```python
from build123d import *

# Parameters (mm, degrees)
SKETCH1_R           = 6
BOSS_EXTRUDE1_DEPTH = 3
SKETCH2_R           = 5.5
BOSS_EXTRUDE2_DEPTH = 0.5
SKETCH3_R           = 6
BOSS_EXTRUDE3_DEPTH = 5
SKETCH4_R           = 1.15
CUT_EXTRUDE1_DEPTH  = 5
SKETCH5_R           = 0.3
BOSS_EXTRUDE4_DEPTH = 5
FILLET1_R           = 0.1
CHAMFER1_SIZE       = 0.05


with BuildPart() as part:
    # Sketch1 → Boss-Extrude1 (new body)
    with BuildSketch(Plane(origin=(0, 0, 0), x_dir=(1, 0, 0), z_dir=(0, 1, 0))):
        with Locations(Location((0, 0, 0), (0, 0, 270))):
            Circle(SKETCH1_R)
    extrude(amount=BOSS_EXTRUDE1_DEPTH)

    # Sketch2 → Boss-Extrude2 (add)
    with BuildSketch(Plane(origin=(0, 3, 0), x_dir=(1, 0, 0), z_dir=(0, 1, 0))):
        with Locations(Location((0, 0, 0), (0, 0, 270))):
            Circle(SKETCH2_R)
    extrude(amount=BOSS_EXTRUDE2_DEPTH)

    # Sketch3 → Boss-Extrude3 (add)
    with BuildSketch(Plane(origin=(0, 3.5, 0), x_dir=(1, 0, 0), z_dir=(0, 1, 0))):
        with Locations(Location((0, 0, 0), (0, 0, 270))):
            Circle(SKETCH3_R)
    extrude(amount=BOSS_EXTRUDE3_DEPTH)

    # Sketch4 → Cut-Extrude1 (cut)
    with BuildSketch(Plane(origin=(0, 8.5, 0), x_dir=(1, 0, 0), z_dir=(0, 1, 0))):
        with Locations(Location((0, 0, 0), (0, 0, 270))):
            Circle(SKETCH4_R)
    extrude(amount=-CUT_EXTRUDE1_DEPTH, mode=Mode.SUBTRACT)

    # Sketch5 → Boss-Extrude4 (add)
    with BuildSketch(Plane.XZ):
        with Locations(Location((-3.25, 0, 0), (0, 0, 90))):
            Circle(SKETCH5_R)
        with Locations(Location((3.25, 0, 0), (0, 0, 90))):
            Circle(SKETCH5_R)
    extrude(amount=BOSS_EXTRUDE4_DEPTH)

    # Fillet1
    fillet1_edges = [part.edges().sort_by_distance(p)[0] for p in [
        (0, 8.5, -6),
        (0, 0, -6),
    ]]
    fillet(fillet1_edges, radius=FILLET1_R)

    # Chamfer1
    chamfer1_edges = [part.edges().sort_by_distance(p)[0] for p in [
        (-3.25, -5, -0.3),
        (3.25, -5, -0.3),
    ]]
    chamfer(chamfer1_edges, length=CHAMFER1_SIZE)


solid = part.part
```
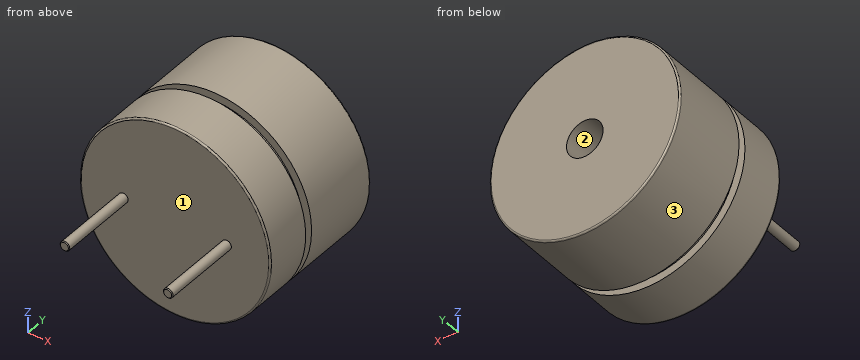
Geometry: final body of the model. Coordinates: model frame, mm. Face numbers are marked on the shaded views. Coordinates: 2 decimals unless noted, no trailing zeros. Order: outer loops, then holes, each group sorted by start corner. A loop starts at its lowest first (then second) coordinate and runs counter-clockwise, first axis right, second up. Notation, with made-up numbers: (6, 24) -> (25, 24) arc R28 cw to (25, 56) -> close; hole circle Ø4 at (16.25, 79.25). An arc over 180 degrees is marked (long way). Write each question's results on one line, items separated by ' | '. Start each with the question number.
1) Cut plane C-C, the plane y = 7.75. Output: boundary loops of the cut face in (x, z), and give its area (3 significant figures).
2) Mould query, pull axis Z, two halves, no side actions, for the marked faces 1, 2 and 3. Classes: released by +Z, released by -Z, zero draft, split by the parting line, or undercut.
3) Cut plane B-B, the plane x = 0. Output: boundary loops of the cut face in (y, z).
4) Material intervals for line 1 along X through (y, z) = (6.75, 0); line 2 along Y through (x, z) = (-4.25, -3.75); line 3 along Y through (x, z) = (-5, -0.75), sorted ascending.
5) First-contact query: pin 1 (5 mm diameter, centred on x = 4.5, y = 3, fed in from +Z); pin 2 (5 mm diameter, centred on x = -3, y = 1.5, fed in from -Z); pin 3 (1.5 mm diameter, centred on x = 2, y = 5.5, fed in from -Z). Flat tips, straight axial feed; report the tip coordinate or a pass-through.
6) Cut plane D-D, the plane y = 2.5. Output: boundary loops of the cut face in (x, z).
Checks:
1) outline: circle Ø12 at (0, 0); hole circle Ø2.3 at (0, 0) | area: 109 mm^2
2) face 1: zero draft | face 2: undercut | face 3: split by the parting line
3) outline: (0, -5.9) arc R0.1 ccw to (0.1, -6) -> (3, -6) -> (3, -5.5) -> (3.5, -5.5) -> (3.5, -6) -> (8.4, -6) arc R0.1 ccw to (8.5, -5.9) -> (8.5, -1.15) -> (3.5, -1.15) -> (3.5, 1.15) -> (8.5, 1.15) -> (8.5, 5.9) arc R0.1 ccw to (8.4, 6) -> (3.5, 6) -> (3.5, 5.5) -> (3, 5.5) -> (3, 6) -> (0.1, 6) arc R0.1 ccw to (0, 5.9) -> close
4) line 1: -6 to -1.15, 1.15 to 6 | line 2: 0 to 3, 3.5 to 8.5 | line 3: 0 to 8.5
5) pin 1: z = 5.66 | pin 2: z = -5.98 | pin 3: z = -5.87
6) outline: circle Ø12 at (0, 0)
